```python
from build123d import *

# Parameters (mm, degrees)
F0_W     = 50.8
F0_H     = 38.1
F0_R     = 9.525
F1_DEPTH = 76.2
F2_SIZE  = 5.08
F3_SIZE  = 5.08
F4_R     = 2.54
F5_T     = 2.54


# Not quite as in the source:
# - a shell that OpenCascade refuses in one call is made with other operations: the cavity is built on its own and cut out


with BuildPart() as f1:
    # F0 (on Front) → F1 (new body)
    with BuildSketch(Plane.XZ):
        with Locations((25.4, 19.05)):
            Rectangle(F0_W, F0_H)
        with Locations((19.05, 19.05)):
            Circle(F0_R, mode=Mode.SUBTRACT)
    extrude(amount=F1_DEPTH)

    # F2
    f2_edges = [f1.edges().sort_by_distance(p)[0] for p in [
        (0, -38.1, 0),
    ]]
    chamfer(f2_edges, length=F2_SIZE)

    # F3
    f3_edges = [f1.edges().sort_by_distance(p)[0] for p in [
        (0, -38.1, 38.1),
        (50.8, -38.1, 38.1),
    ]]
    chamfer(f3_edges, length=F3_SIZE)

    # F4
    f4_edges = [f1.edges().sort_by_distance(p)[0] for p in [
        (0, -76.2, 19.05),
        (2.54, -76.2, 35.56),
        (2.54, -76.2, 2.54),
        (25.4, -76.2, 38.1),
        (27.94, -76.2, 0),
        (48.26, -76.2, 35.56),
        (50.8, -76.2, 16.51),
        (9.525, -76.2, 19.05),
    ]]
    fillet(f4_edges, radius=F4_R)

    # F5: shell of thickness 2.54, made by hand


with BuildPart() as f5_core1:
    # F5_t2: copy of F1
    add(f1.part)

    # the walls: a layer under each face that stays
    f5_faces = [f5_core1.faces().sort_by_distance(p)[0] for p in [
        (0, -36.83, 19.05),
        (2.54, -36.83, 35.56),
        (2.54, -36.83, 2.54),
        (25.4, -36.83, 38.1),
        (10.16, -76.2, 8.0433333333),
        (27.94, -36.83, 0),
        (48.26, -36.83, 35.56),
        (50.8, -36.83, 16.51),
        (9.525, -36.83, 19.05),
    ]]
    thicken(f5_faces, amount=-F5_T, mode=Mode.SUBTRACT)


with BuildPart() as f1_1:
    add(f1.part)

    # what is left inside the walls is the cavity
    f5_cavity = [f5_core1.part.solids().sort_by_distance(p)[0] for p in [
        (6.9596, -49.106667, 19.05),
    ]]
    add(f5_cavity, mode=Mode.SUBTRACT)


solid = f1_1.part
```
The model under review builds one solid part; all positions refer to its coordinate system, in mm. A direction names the side the tool comes from. Give positions to 0.01 mm unless a question says otherwise; leave off trailing zeros. Write each loop counter-clockwise with the first axis right and the second up, starting at its lowest first coordinate (ties: lowest second). Pieces come first, ordered by that corner, then holes. Notation, with made-up numbers: M 55.5,21 L 67.5,21 A26 ccw 67.5,43 Z; hole C 1,63.5 d3. An arc over 180 degrees is marked long. Write item = value, one per line. Start each with the question number.
Q1. We need section D-D (x = 36). State the section outline as (y, z) points.
Q2. We need section A-A (y = -9). State the section outline as (x, z) points (3 decimals), plus the area to 3 significant figures.
Q3. Mouldability with a two-part tool opening along Z and no side actions: class faces 1 (the face through (35, -73.66, 19)), 2 (the face through (4.36, -36.31, 4.31)), 3 (the face through (0.724, -75.436, 19.246)), 4 (the face through (28.26, -75.476, 0.764)) as released by +Z, released by -Z, zero draft, split by the parting line, or undercut.
Q4. We need section C-C (x = 19.05). State the section outline as (y, z) points (3 decimals), plus the area to 3 significant figures.
Q5. Machinability: for faces 5 (the face through (2.58, -36.31, 35.6)), 6 (the face through (48.26, -36, 17)), which of the approach directions +Z, -Z, +X, -X, +Y, -Y give a long, thin tool a straight path to every point of the face, cutting with its end or side? Answer none if there is none.
Q6. Clearance check with flat-ended pins moving along their axes: pin 1 (4 mm diameter, centred on x = 25, z = 10, fed in from +Y); pin 2 (1 mm diameter, centred on x = 27, z = 32.5, fed in from +Y); pin 3 (2 mm diameter, centred on x = 15, z = 28, fed in from -Y). State where each tip first meets the part, or that it passes through.
Q7. For line 1 (Z direction, x = 19, y = -22); line 2 (X direction, y = -22, z = 19); line 3 (Z direction, x = 32, y = -33), list the stretches that pass through material, from the lowest coordinate up.
Q8. We need section B-B (z = 19.05). State the section outline as (x, y) points (3 decimals).
Result set:
q1.outline = M -76.2,2.54 A2.54 ccw -73.66,0 L 0,0 L 0,2.54 L -73.66,2.54 L -73.66,35.56 L 0,35.56 L 0,38.1 L -73.66,38.1 A2.54 ccw -76.2,35.56 Z
q2.outline = M 0,5.08 L 5.08,0 L 50.8,0 L 50.8,33.02 L 45.72,38.1 L 5.08,38.1 L 0,33.02 Z; C 19.05,19.05 d24.13; hole M 2.54,6.132 L 6.132,2.54 L 48.26,2.54 L 48.26,31.968 L 44.668,35.56 L 6.132,35.56 L 2.54,31.968 Z; hole C 19.05,19.05 d19.05
q2.area = 579 mm2
q3.face_1 = undercut
q3.face_2 = undercut
q3.face_3 = zero draft
q3.face_4 = released by -Z
q4.outline = M -76.2,2.54 A2.54 ccw -73.66,0 L 0,0 L 0,2.54 L -73.66,2.54 L -73.66,6.985 L 0,6.985 L 0,9.525 L -73.66,9.525 A2.54 ccw -76.2,6.985 Z; M -76.2,31.115 A2.54 ccw -73.66,28.575 L 0,28.575 L 0,31.115 L -73.66,31.115 L -73.66,35.56 L 0,35.56 L 0,38.1 L -73.66,38.1 A2.54 ccw -76.2,35.56 Z
q4.area = 791 mm2
q5.face_5 = +Z, -X, +Y, -Y
q5.face_6 = +Y
q6.pin_1 = 0
q6.pin_2 = -73.66
q6.pin_3 = -75.88
q7.line_1 = 0 to 2.54, 6.99 to 9.53, 28.57 to 31.11, 35.56 to 38.1
q7.line_2 = 0 to 2.54, 6.99 to 9.53, 28.57 to 31.11, 48.26 to 50.8
q7.line_3 = 0 to 2.54, 35.56 to 38.1
q8.outline = M 0,-73.66 A2.54 ccw 2.54,-76.2 L 6.985,-76.2 A2.54 ccw 9.525,-73.66 L 9.525,0 L 6.985,0 L 6.985,-73.66 L 2.54,-73.66 L 2.54,0 L 0,0 Z; M 28.575,-73.66 A2.54 ccw 31.115,-76.2 L 48.26,-76.2 A2.54 ccw 50.8,-73.66 L 50.8,0 L 48.26,0 L 48.26,-73.66 L 31.115,-73.66 L 31.115,0 L 28.575,0 Z
